The model under review builds one solid part; all positions refer to its coordinate system, in mm. A direction names the side the tool comes from. Coordinates: 2 decimals unless noted, no trailing zeros. Order: outer loops, then holes, each group sorted by start corner. A loop starts at its lowest first (then second) coordinate and runs counter-clockwise, first axis right, second up. Notation, with made-up numbers: (-29, -35) -> (-18, -35) arc R14 ccw to (-18, -18) -> close; hole circle Ø3 at (-6.5, -18). An arc over 180 degrees is marked (long way). Use one line per item in the form item = value.
from build123d import *

# Parameters (mm, degrees)
CUT_EXTRUDE2_START  = -31.75
CUT_EXTRUDE2_DEPTH  = 31.75
CIRPATTERN1_COUNT   = 6
CUT_EXTRUDE3_DEPTH  = 31.75
CIRPATTERN2_COUNT   = 6
CUT_EXTRUDE4_START  = -12.7
SKETCH7_R           = 25.4
SKETCH7_R_2         = 22.225
CUT_EXTRUDE4_DEPTH  = 12.7
SKETCH8_R           = 25.4
SKETCH8_R_2         = 22.225
CUT_EXTRUDE5_DEPTH  = 12.7
BOSS_EXTRUDE1_START = -38.1
SKETCH9_R           = 34.925
BOSS_EXTRUDE1_DEPTH = 12.7
BOSS_EXTRUDE2_START = 76.2
SKETCH10_R          = 22.225
BOSS_EXTRUDE2_DEPTH = 76.2


with BuildPart() as part:
    # Sketch3 → Revolve1 (revolve)
    with BuildSketch(Plane(origin=(0, 0, 0), x_dir=(0, 0, -1), z_dir=(1, 0, 0)), mode=Mode.PRIVATE) as revolve1_sk:
        Polygon((-146.05, 0), (-146.05, 25.4), (-88.9, 25.4), (-88.9, 28.575), (-57.15, 28.575), (-57.15, 31.75), (44.45, 31.75), (44.45, 28.575), (76.2, 28.575), (76.2, 25.4), (146.05, 25.4), (146.05, 0), align=None)
    revolve(revolve1_sk.sketch.rotate(Axis((0, 0, 128.279136691), (0, 0, -1)), 90), axis=Axis((0, 0, 128.279136691), (0, 0, -1)))

    # Sketch5 → Cut-Extrude2 (cut)
    with BuildSketch(Plane.XY.offset(88.9).offset(CUT_EXTRUDE2_START)):
        with BuildLine():
            Line((0, 28.575), (0, 25.4))
            ThreePointArc((0, 25.4), (3.315365282, 25.182699479), (6.574003746, 24.534515988))
            Line((6.574003746, 24.534515988), (7.395754214, 27.601330486))
            ThreePointArc((7.395754214, 27.601330486), (3.729785943, 28.330536914), (0, 28.575))
        make_face()
        with BuildLine():
            ThreePointArc((-6.574003746, 24.534515988), (-3.315365282, 25.182699479), (0, 25.4))
            Line((0, 25.4), (0, 28.575))
            ThreePointArc((0, 28.575), (-3.729785943, 28.330536914), (-7.395754214, 27.601330486))
            Line((-7.395754214, 27.601330486), (-6.574003746, 24.534515988))
        make_face()
    cut_extrude2 = extrude(amount=CUT_EXTRUDE2_DEPTH, mode=Mode.SUBTRACT)

    # CirPattern1: Cut-Extrude2 ×6 about axis
    cirpattern1_axis = Axis((0, 0, 0), (0, 0, 1))
    for i in range(1, CIRPATTERN1_COUNT):
        add(cut_extrude2.rotate(cirpattern1_axis, i * 360 / CIRPATTERN1_COUNT), mode=Mode.SUBTRACT)

    # Sketch6 → Cut-Extrude3 (cut)
    with BuildSketch(Plane(origin=(0, 0, -76.2), x_dir=(-1, 0, 0), z_dir=(0, 0, -1))):
        with BuildLine():
            Line((0, 28.575), (0, 25.4))
            ThreePointArc((0, 25.4), (3.315365282, 25.182699479), (6.574003746, 24.534515988))
            Line((6.574003746, 24.534515988), (7.395754214, 27.601330486))
            ThreePointArc((7.395754214, 27.601330486), (3.729785943, 28.330536914), (0, 28.575))
        make_face()
        with BuildLine():
            ThreePointArc((-6.574003746, 24.534515988), (-3.315365282, 25.182699479), (0, 25.4))
            Line((0, 25.4), (0, 28.575))
            ThreePointArc((0, 28.575), (-3.729785943, 28.330536914), (-7.395754214, 27.601330486))
            Line((-7.395754214, 27.601330486), (-6.574003746, 24.534515988))
        make_face()
    cut_extrude3 = extrude(amount=-CUT_EXTRUDE3_DEPTH, mode=Mode.SUBTRACT)

    # CirPattern2: Cut-Extrude3 ×6 about axis
    cirpattern2_axis = Axis((0, 0, 0), (0, 0, 1))
    for i in range(1, CIRPATTERN2_COUNT):
        add(cut_extrude3.rotate(cirpattern2_axis, i * 360 / CIRPATTERN2_COUNT), mode=Mode.SUBTRACT)

    # Sketch7 → Cut-Extrude4 (cut)
    with BuildSketch(Plane.XY.offset(146.05).offset(CUT_EXTRUDE4_START)):
        Circle(SKETCH7_R)
        Circle(SKETCH7_R_2, mode=Mode.SUBTRACT)
    extrude(amount=CUT_EXTRUDE4_DEPTH, mode=Mode.SUBTRACT)

    # Sketch8 → Cut-Extrude5 (cut)
    with BuildSketch(Plane(origin=(0, 0, -146.05), x_dir=(-1, 0, 0), z_dir=(0, 0, -1))):
        with Locations(Location((0, 0, 0), (0, 0, 195))):
            Circle(SKETCH8_R)
        with Locations(Location((0, 0, 0), (0, 0, 180))):
            Circle(SKETCH8_R_2, mode=Mode.SUBTRACT)
    extrude(amount=-CUT_EXTRUDE5_DEPTH, mode=Mode.SUBTRACT)

    # Sketch9 → Boss-Extrude1 (add)
    with BuildSketch(Plane.XY.offset(57.15).offset(BOSS_EXTRUDE1_START)):
        Circle(SKETCH9_R)
    extrude(amount=-BOSS_EXTRUDE1_DEPTH)

    # Sketch10 → Boss-Extrude2 (add)
    with BuildSketch(Plane(origin=(0, 0, -146.05), x_dir=(-1, 0, 0), z_dir=(0, 0, -1)).offset(BOSS_EXTRUDE2_START)):
        Circle(SKETCH10_R)
    extrude(amount=-BOSS_EXTRUDE2_DEPTH)


solid = part.part
Item 1: Tool access review of faces 1 (the face through (13, -23, 88.9)), 2 (the face through (-28.575, -0.105, 72.803)), 3 (the face through (21.199, 6.676, 139.611)), 4 (the face through (-28.575, -0.105, -60.547)): name each direction out of +Z, -Z, +X, -X, +Y, -Y from which nothing blocks a thin tool from reaching the whole face with its end or side.
Results found:
face_1 = +Z, +X, -Y
face_2 = +Z, -X
face_3 = +Z
face_4 = -Z, -X
Item 2: We need section C-C (z = -10.5). Write out the cut boundary in (x, y).
Results found:
outline = circle Ø63.5 at (0, 0)
Item 3: We need section B-B (z = -110.5). Write out the cut boundary in (x, y).
Results found:
outline = circle Ø50.8 at (0, 0)
Item 4: We need section A-A (z = -54). Write out the cut boundary in (x, y) (3 decimals).
Results found:
outline = (-27.601, -7.396) -> (-24.535, -6.574) arc R25.4 ccw to (-17.961, -17.961) -> (-20.206, -20.206) arc R28.575 ccw to (-7.396, -27.601) -> (-6.574, -24.535) arc R25.4 ccw to (6.574, -24.535) -> (7.396, -27.601) arc R28.575 ccw to (20.206, -20.206) -> (17.961, -17.961) arc R25.4 ccw to (24.535, -6.574) -> (27.601, -7.396) arc R28.575 ccw to (27.601, 7.396) -> (24.535, 6.574) arc R25.4 ccw to (17.961, 17.961) -> (20.206, 20.206) arc R28.575 ccw to (7.396, 27.601) -> (6.574, 24.535) arc R25.4 ccw to (-6.574, 24.535) -> (-7.396, 27.601) arc R28.575 ccw to (-20.206, 20.206) -> (-17.961, 17.961) arc R25.4 ccw to (-24.535, 6.574) -> (-27.601, 7.396) arc R28.575 ccw to start
Item 5: Clearance check with flat-ended pins moving along their axes: pin 1 (3 mm diameter, centred on x = -26.5, y = 2.5, fed in from +Z); pin 2 (1.2 mm diameter, centred on x = 26.5, y = 0.5, fed in from -Z); pin 3 (4 mm diameter, centred on x = -25.5, z = -12, fed in from +Y). State where each tip first meets the part, or that it passes through.
Results found:
pin_1 = 133.35
pin_2 = -76.2
pin_3 = 21.35
Item 6: To check wall thickness, follow L1, parallel to Y at x = 20, z = 80; L2, parallel to X at y = 13, z = -140; L3, parallel to Z at x = -8.5, y = 24.5. State the ranges of each line that lie inside material, in increasing order. Write a range as from..to.
Results found:
L1 = -20.41..-20, -15.66..15.66, 20..20.41
L2 = -18.03..18.03
L3 = -76.2..88.9
